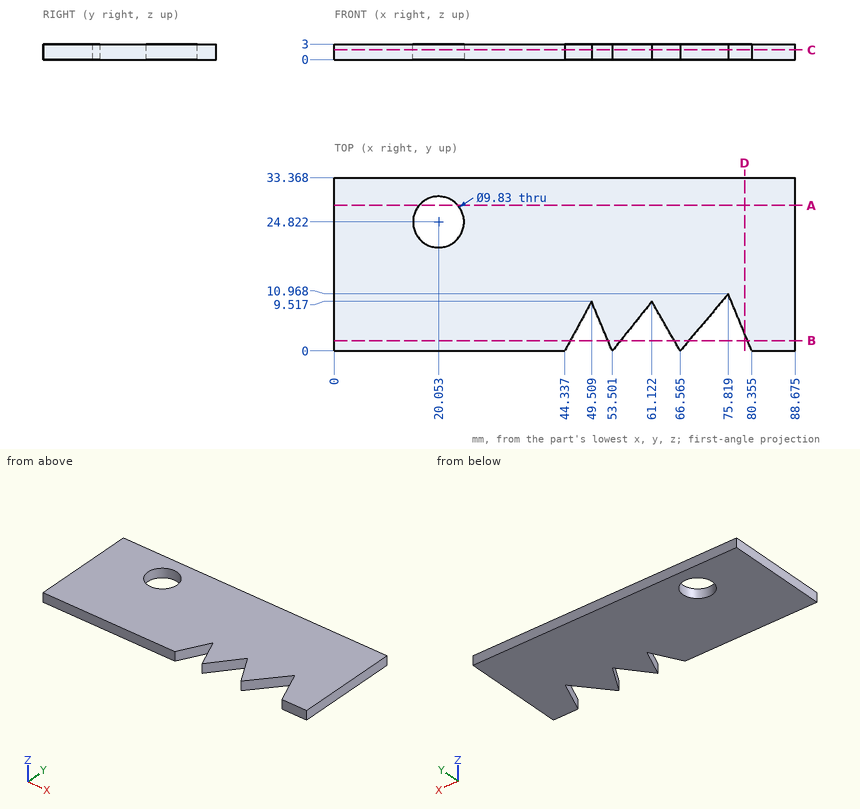
Geometry: see drawing. Coordinates: mm, zero at the bounding-box minimum. Coordinates: 2 decimals unless noted, no trailing zeros. Loops run counter-clockwise (first coordinate to the right, second up) from the corner with the lowest first, then second, coordinate; pieces in that order, holes last. Notation, with made-up numbers: (87.25, 33.25) - (113.25, 33.25) arc R21 cw to (113.25, 50.25) - close; hole circle Ø9 at (4, 46.5). An arc over 180 degrees is marked (long way). Put each result on its own line as item: value. Start each with the question number.
Q1. Cut plane A-A, the plane y = 28. Return loops of the section in (x, z) (1 decimal).
Q2. Cut plane D-D, the plane x = 79. Return loops of the section in (y, z).
Q3. Pin query (flat end, axial travel): pin 1 Ø6 at (x, y) = (20.05, 24.82) entering from -Z. Return the tip coordinate at first contact, or that it passes through.
Q4. Cut plane B-B, the plane y = 2. Return loops of the section in (x, z) (1 decimal).
Q5. Line query: line 1 (X direction, y = 4, z = 1.8) (1 decimal); line 2 (X direction, y = 7.5, z = 2.25) (1 decimal); line 3 (X direction, y = 27, z = 1.55) (1 decimal). Output: solid intervals per line, ascending.
Q6. Cut plane C-C, the plane z = 1.85. Return loops of the section in (x, y) (1 decimal).
Filled sheet:
1. outline: (0, 0) - (16.3, 0) - (16.3, 3) - (0, 3) - close; (23.8, 0) - (88.7, 0) - (88.7, 3) - (23.8, 3) - close
2. outline: (3.28, 0) - (33.37, 0) - (33.37, 3) - (3.28, 3) - close
3. pin 1: through
4. outline: (0, 0) - (45.4, 0) - (45.4, 3) - (0, 3) - close; (52.7, 0) - (55.1, 0) - (55.1, 3) - (52.7, 3) - close; (65.4, 0) - (68.3, 0) - (68.3, 3) - (65.4, 3) - close; (79.5, 0) - (88.7, 0) - (88.7, 3) - (79.5, 3) - close
5. line 1: 0 to 46.5, 51.8 to 56.7, 64.3 to 69.9, 78.7 to 88.7
5. line 2: 0 to 48.4, 50.4 to 59.5, 62.3 to 72.9, 77.3 to 88.7
5. line 3: 0 to 15.6, 24.5 to 88.7
6. outline: (0, 0) - (44.3, 0) - (49.5, 9.5) - (53.5, 0) - (61.1, 9.5) - (66.6, 0) - (75.8, 11) - (80.4, 0) - (88.7, 0) - (88.7, 33.4) - (0, 33.4) - close; hole circle Ø9.8 at (20.1, 24.8)
